Read the model definition and answer for the solid it produces. Units are mm, in the model's axes. Face numbers are marked on the shaded views. A direction names the side the tool comes from. Round coordinates to 2 decimals unless told otherwise and drop trailing zeros. Order: outer loops, then holes, each group sorted by start corner. A loop starts at its lowest first (then second) coordinate and runs counter-clockwise, first axis right, second up. Notation, with made-up numbers: (30, 65.25) -> (68, 65.25) arc R19 cw to (68, 74.25) -> close; hole circle Ø5 at (74.25, -26.5). An arc over 180 degrees is marked (long way). Use a Markdown table: item, result. Add a question column.
1. Section C-C, the plane x = -5 is taken. Give the vertices of the cut face in (y, z), then the cut area to 3 significant figures.
2. Consider L1, parallel to Y at x = -10.5, z = 5.25; L2, parallel to Z at x = 15, y = 3.5; L3, parallel to X at y = 22, z = 28.75. Determine where each line is inside the solid, lowest interval first. Write a range as [from, to].
3. The mould has two halves that part along X. Classify the marked faces 4, 5, 6 and 7: +X half, -X half, draft (parallel to the pull), parting line (faces both ways), or undercut.
4. Section B-B, the plane z = 15.75 is taken. Give the vertices of the cut face in (x, y).
5. Section A-A, the plane y = 20.5 is taken. Give the vertices of the cut face in (x, z).
6. Given pin 1 (2 mm diameter, centred on x = 28.5, z = 4.5, fed in from +Y); pin 2 (1.5 mm diameter, centred on x = 12, z = 16, fed in from +Y); pin 3 (9 mm diameter, centred on x = 29, y = 16, fed in from +Z), each flat-ended and moving along its own axis, determine where each tip first touches the part or whether it passes through.
7. For the marked faces 1, 2 and 3, determine the directions among +Z, -Z, +X, -X, +Y, -Y from which every point of the face is accessible in a straight line to the end or side of a thin tool.
8. Section D-D, the plane y = 14 is taken. Give the vertices of the cut face in (x, z).
```python
from build123d import *

# Parameters (mm, degrees)
F0_W     = 55
F0_H     = 30
F1_DEPTH = 30
F2_W     = 30
F2_H     = 15
F3_DEPTH = 30.001
F5_DEPTH = 5


with BuildPart() as f1:
    # F0 (on Top) → F1 (new body)
    with BuildSketch(Plane.XY):
        with Locations((9.0955648875, 9.9145695567)):
            Rectangle(F0_W, F0_H)
    extrude(amount=F1_DEPTH)

    # F2 (on face) → F3 (cut, through all)
    with BuildSketch(Plane(origin=(0, 24.9145695567, 0), x_dir=(-1, 0, 0), z_dir=(0, 1, 0))):
        with Locations((-21.5955648875, 22.5)):
            Rectangle(F2_W, F2_H)
    extrude(amount=-F3_DEPTH, mode=Mode.SUBTRACT)

    # F4 (on face) → F5 (cut)
    with BuildSketch(Plane(origin=(0, 24.9145695567, 0), x_dir=(-1, 0, 0), z_dir=(0, 1, 0))):
        with BuildLine():
            Line((-34.0955648875, 0), (-19.0955648875, 0))
            ThreePointArc((-19.0955648875, 0), (-26.5955648875, 7.5), (-34.0955648875, 0))
        make_face()
        with BuildLine():
            ThreePointArc((15.9044351125, 0), (8.4044351125, 7.5), (0.9044351125, 0))
            Line((0.9044351125, 0), (15.9044351125, 0))
        make_face()
    extrude(amount=-F5_DEPTH, mode=Mode.SUBTRACT)


solid = f1.part
```
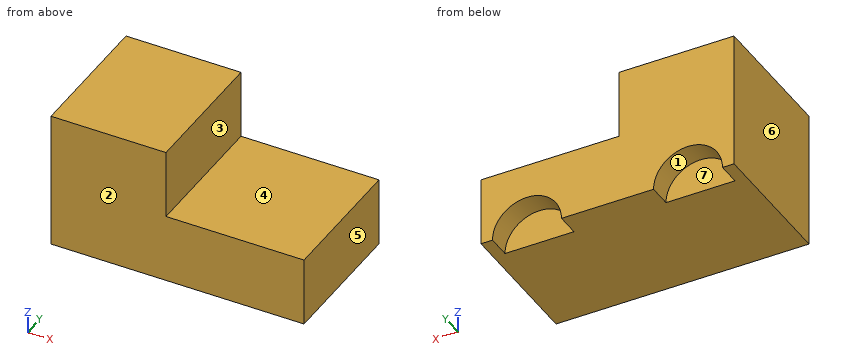
Verdict:
| question | item | result |
|---|---|---|
| 1 | outline | (-5.09, 0) -> (19.91, 0) -> (19.91, 6.68) -> (24.91, 6.68) -> (24.91, 30) -> (-5.09, 30) -> close |
| 1 | area | 867 mm2 |
| 2 | L1 | y = [-5.09, 19.91] |
| 2 | L2 | z = [0, 15] |
| 2 | L3 | x = [-18.4, 6.6] |
| 3 | face 4 | draft |
| 3 | face 5 | +X half |
| 3 | face 6 | -X half |
| 3 | face 7 | undercut |
| 4 | outline | (-18.4, -5.09) -> (6.6, -5.09) -> (6.6, 24.91) -> (-18.4, 24.91) -> close |
| 5 | outline | (-18.4, 0) -> (-15.9, 0) arc R7.5 cw to (-0.9, 0) -> (19.1, 0) arc R7.5 cw to (34.1, 0) -> (36.6, 0) -> (36.6, 15) -> (6.6, 15) -> (6.6, 30) -> (-18.4, 30) -> close |
| 6 | pin 1 | stops at y = 19.91 |
| 6 | pin 2 | passes through |
| 6 | pin 3 | stops at z = 15 |
| 7 | face 1 | -Z, +Y |
| 7 | face 2 | +Z, -Z, +X, -X, -Y |
| 7 | face 3 | +Z, +X, +Y, -Y |
| 8 | outline | (-18.4, 0) -> (36.6, 0) -> (36.6, 15) -> (6.6, 15) -> (6.6, 30) -> (-18.4, 30) -> close |
